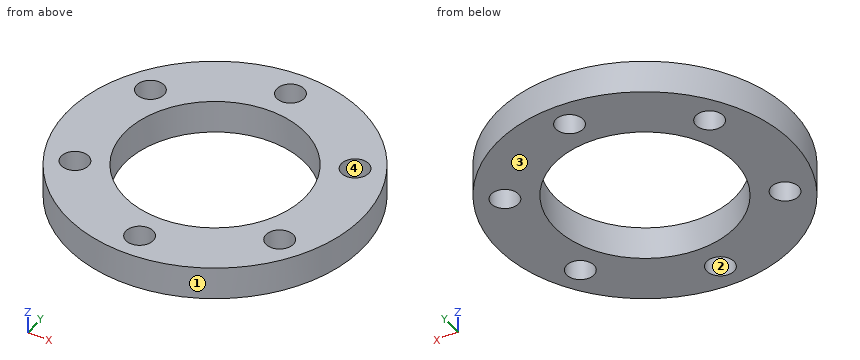
Autodesk Inventor part; units mm, degrees
ref_plane "YZ Plane" through (0, 0, 0) normal (1, 0, 0) x (0, 1, 0)
ref_plane "XZ Plane" through (0, 0, 0) normal (0, 1, 0) x (-1, 0, 0)
ref_plane "XY Plane" through (0, 0, 0) normal (0, 0, 1) x (1, 0, 0)
sketch "Sketch1" plane through (0, 0, 0) normal (0, 0, 1) x (1, 0, 0)
  circle A0 centre (0, 0) radius 16.5
  circle A1 centre (0, 0) radius 27
  point P0 (0, 22)
  point P1 (-19.0526, 11)
  point P2 (-19.0526, -11)
  point P3 (0, -22)
  point P4 (19.0526, -11)
  point P5 (19.0526, 11)
  dimension "d9" = 33
  dimension "d20" = 22
  dimension "d23" = 360
  dimension "d58" = 54
extrude "Extrusion2" add sketch "Sketch1" along normal blind 6
hole "Hole3" at (0, 22, 0) at (-19.0526, 11, 0) at (-19.0526, -11, 0) at (0, -22, 0) at (19.0526, 11, 0) at (19.0526, -11, 0) direction (0, 0, 1) diameter 5 end through all
properties part number "SpacerSprocketHubPlate"
Geometry check sheet. Reference: the model listing, model coordinates, mm. Face numbers are marked on the shaded views. Coordinates: 2 decimals unless noted, no trailing zeros. Loops run counter-clockwise (first coordinate to the right, second up) from the corner with the lowest first, then second, coordinate; pieces in that order, holes last. Notation, with made-up numbers: (-30, -9.75) - (-10, -9.75) arc R10 ccw to (-10, -4.75) - close; hole circle Ø3 at (6.5, 85.5). An arc over 180 degrees is marked (long way). One line per item, written item: value. Start each with the question number.
(1) Mould release check, pull along X, two halves, no side actions. Record for the marked faces 1, 2, 3 and 4: released by +X, released by -X, zero draft, split by the parting line, or undercut.
(2) Cross-section at C-C on x = 0. Enter the section's corners in (y, z).
(3) Depth check by flat-ended pin: P1, Ø4, axis at x = -19.05, y = 11, coming from the -Z side; P2, Ø6, axis at x = -19.05, y = -11, coming from the -Z side; P3, Ø3, axis at x = 5, z = 3, coming from the +Y side; P4, Ø3, axis at x = 0, z = 1, coming from the +Y side. Enter the tip coordinate at first touch or a pass-through.
(4) Cross-section at B-B on x = -11.5. Enter the section's corners in (y, z), plus the area to 3 significant figures.
(5) Cross-section at D-D on y = 11. Enter the section's corners in (x, z).
(6) Material ranges on line 1 (Y direction, x = 0, z = 1.6); line 2 (X direction, y = 11, z = 1.65); line 3 (Y direction, x = -18, z = 4.6), recorded low to high. Write a range as [from, to].
(7) Cross-section at A-A on y = 0. Enter the section's corners in (x, z).
Results below:
1. face 1: split by the parting line
1. face 2: undercut
1. face 3: zero draft
1. face 4: undercut
2. outline: (-27, 0) - (-24.5, 0) - (-24.5, 6) - (-27, 6) - close; (-19.5, 0) - (-16.5, 0) - (-16.5, 6) - (-19.5, 6) - close; (16.5, 0) - (19.5, 0) - (19.5, 6) - (16.5, 6) - close; (24.5, 0) - (27, 0) - (27, 6) - (24.5, 6) - close
3. P1: passes through
3. P2: stops at z = 0
3. P3: stops at y = 26.77
3. P4: stops at y = 27
4. outline: (-24.43, 0) - (-11.83, 0) - (-11.83, 6) - (-24.43, 6) - close; (11.83, 0) - (24.43, 0) - (24.43, 6) - (11.83, 6) - close
4. area: 151 mm2
5. outline: (-24.66, 0) - (-21.55, 0) - (-21.55, 6) - (-24.66, 6) - close; (-16.55, 0) - (-12.3, 0) - (-12.3, 6) - (-16.55, 6) - close; (12.3, 0) - (16.55, 0) - (16.55, 6) - (12.3, 6) - close; (21.55, 0) - (24.66, 0) - (24.66, 6) - (21.55, 6) - close
6. line 1: y = [-27, -24.5], [-19.5, -16.5], [16.5, 19.5], [24.5, 27]
6. line 2: x = [-24.66, -21.55], [-16.55, -12.3], [12.3, 16.55], [21.55, 24.66]
6. line 3: y = [-20.12, -13.27], [-8.73, 8.73], [13.27, 20.12]
7. outline: (-27, 0) - (-16.5, 0) - (-16.5, 6) - (-27, 6) - close; (16.5, 0) - (27, 0) - (27, 6) - (16.5, 6) - close
